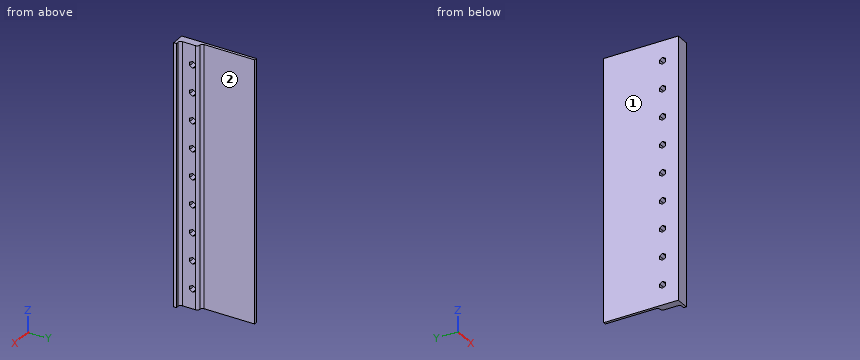
from build123d import *

# Parameters (mm, degrees)
GENERAL_EXTRUDE_DEPTH       = 925
ROUNDING_R                  = 5
ROLLER_HOLDERS_DEPTH        = 926.55388822
SKETCH5_W                   = 5
SKETCH5_H                   = 1850
GUARD_RAIL_DEPTH            = 100
GUARD_RAIL_SUPPORT_FILLET_R = 5
CUT_TO_SIZE_DEPTH           = 934.086276825
CUT_TO_SIZE_DEPTH_BACK      = 934.086276825
SKETCH6_W                   = 1357.48
SKETCH6_H                   = 140


with BuildPart() as part:
    # Sketch2 → General extrude (new, symmetric)
    with BuildSketch(Plane.XY):
        Polygon((-12.5, 20), (-12.5, -20), (12.5, -20), (12.5, -15), (2.5, -15), (2.5, 20), align=None)
    extrude(amount=GENERAL_EXTRUDE_DEPTH, both=True)

    # Rounding
    rounding_edges = [part.edges().sort_by_distance(p)[0] for p in [
        (2.5, 20, 0),
        (2.5, -15, 0),
    ]]
    fillet(rounding_edges, radius=ROUNDING_R)

    # Sketch3 → Roller holders (cut, through all)
    with BuildSketch(Plane.ZY.offset(12.5)):
        Polygon((-884.3762927, 3.8875), (-881.168390267, 9.44375), (-884.3762927, 15), (-890.792097567, 15), (-894, 9.44375), (-890.792097567, 3.8875), align=None)
        Polygon((-832.165457693, 3.8875), (-828.957555259, 9.44375), (-832.165457693, 15), (-838.581262559, 15), (-841.789164992, 9.44375), (-838.581262559, 3.8875), align=None)
        Polygon((-779.954622685, 3.8875), (-776.746720252, 9.44375), (-779.954622685, 15), (-786.370427551, 15), (-789.578329984, 9.44375), (-786.370427551, 3.8875), align=None)
        Polygon((-727.743787677, 3.8875), (-724.535885244, 9.44375), (-727.743787677, 15), (-734.159592543, 15), (-737.367494976, 9.44375), (-734.159592543, 3.8875), align=None)
        Polygon((-675.532952669, 3.8875), (-672.325050236, 9.44375), (-675.532952669, 15), (-681.948757535, 15), (-685.156659969, 9.44375), (-681.948757535, 3.8875), align=None)
        Polygon((-623.322117661, 3.8875), (-620.114215228, 9.44375), (-623.322117661, 15), (-629.737922528, 15), (-632.945824961, 9.44375), (-629.737922528, 3.8875), align=None)
        Polygon((-571.111282653, 3.8875), (-567.90338022, 9.44375), (-571.111282653, 15), (-577.52708752, 15), (-580.734989953, 9.44375), (-577.52708752, 3.8875), align=None)
        Polygon((-518.900447645, 3.8875), (-515.692545212, 9.44375), (-518.900447645, 15), (-525.316252512, 15), (-528.524154945, 9.44375), (-525.316252512, 3.8875), align=None)
        Polygon((-466.689612638, 3.8875), (-463.481710204, 9.44375), (-466.689612638, 15), (-473.105417504, 15), (-476.313319937, 9.44375), (-473.105417504, 3.8875), align=None)
        Polygon((-414.47877763, 3.8875), (-411.270875197, 9.44375), (-414.47877763, 15), (-420.894582496, 15), (-424.102484929, 9.44375), (-420.894582496, 3.8875), align=None)
        Polygon((-362.267942622, 3.8875), (-359.060040189, 9.44375), (-362.267942622, 15), (-368.683747488, 15), (-371.891649921, 9.44375), (-368.683747488, 3.8875), align=None)
        Polygon((-310.057107614, 3.8875), (-306.849205181, 9.44375), (-310.057107614, 15), (-316.47291248, 15), (-319.680814914, 9.44375), (-316.47291248, 3.8875), align=None)
        Polygon((-257.846272606, 3.8875), (-254.638370173, 9.44375), (-257.846272606, 15), (-264.262077472, 15), (-267.469979906, 9.44375), (-264.262077472, 3.8875), align=None)
        Polygon((-205.635437598, 3.8875), (-202.427535165, 9.44375), (-205.635437598, 15), (-212.051242465, 15), (-215.259144898, 9.44375), (-212.051242465, 3.8875), align=None)
        Polygon((-153.42460259, 3.8875), (-150.216700157, 9.44375), (-153.42460259, 15), (-159.840407457, 15), (-163.04830989, 9.44375), (-159.840407457, 3.8875), align=None)
        Polygon((-101.213767583, 3.8875), (-98.005865149, 9.44375), (-101.213767583, 15), (-107.629572449, 15), (-110.837474882, 9.44375), (-107.629572449, 3.8875), align=None)
        Polygon((-49.002932575, 3.8875), (-45.795030141, 9.44375), (-49.002932575, 15), (-55.418737441, 15), (-58.626639874, 9.44375), (-55.418737441, 3.8875), align=None)
        Polygon((3.207902433, 3.8875), (6.415804866, 9.44375), (3.207902433, 15), (-3.207902433, 15), (-6.415804866, 9.44375), (-3.207902433, 3.8875), align=None)
        Polygon((55.418737441, 3.8875), (58.626639874, 9.44375), (55.418737441, 15), (49.002932575, 15), (45.795030141, 9.44375), (49.002932575, 3.8875), align=None)
        Polygon((107.629572449, 3.8875), (110.837474882, 9.44375), (107.629572449, 15), (101.213767583, 15), (98.005865149, 9.44375), (101.213767583, 3.8875), align=None)
        Polygon((159.840407457, 3.8875), (163.04830989, 9.44375), (159.840407457, 15), (153.42460259, 15), (150.216700157, 9.44375), (153.42460259, 3.8875), align=None)
        Polygon((212.051242465, 3.8875), (215.259144898, 9.44375), (212.051242465, 15), (205.635437598, 15), (202.427535165, 9.44375), (205.635437598, 3.8875), align=None)
        Polygon((264.262077472, 3.8875), (267.469979906, 9.44375), (264.262077472, 15), (257.846272606, 15), (254.638370173, 9.44375), (257.846272606, 3.8875), align=None)
        Polygon((316.47291248, 3.8875), (319.680814914, 9.44375), (316.47291248, 15), (310.057107614, 15), (306.849205181, 9.44375), (310.057107614, 3.8875), align=None)
        Polygon((368.683747488, 3.8875), (371.891649921, 9.44375), (368.683747488, 15), (362.267942622, 15), (359.060040189, 9.44375), (362.267942622, 3.8875), align=None)
        Polygon((420.894582496, 3.8875), (424.102484929, 9.44375), (420.894582496, 15), (414.47877763, 15), (411.270875197, 9.44375), (414.47877763, 3.8875), align=None)
        Polygon((473.105417504, 3.8875), (476.313319937, 9.44375), (473.105417504, 15), (466.689612638, 15), (463.481710204, 9.44375), (466.689612638, 3.8875), align=None)
        Polygon((525.316252512, 3.8875), (528.524154945, 9.44375), (525.316252512, 15), (518.900447645, 15), (515.692545212, 9.44375), (518.900447645, 3.8875), align=None)
        Polygon((577.52708752, 3.8875), (580.734989953, 9.44375), (577.52708752, 15), (571.111282653, 15), (567.90338022, 9.44375), (571.111282653, 3.8875), align=None)
        Polygon((629.737922528, 3.8875), (632.945824961, 9.44375), (629.737922528, 15), (623.322117661, 15), (620.114215228, 9.44375), (623.322117661, 3.8875), align=None)
        Polygon((681.948757535, 3.8875), (685.156659969, 9.44375), (681.948757535, 15), (675.532952669, 15), (672.325050236, 9.44375), (675.532952669, 3.8875), align=None)
        Polygon((734.159592543, 3.8875), (737.367494976, 9.44375), (734.159592543, 15), (727.743787677, 15), (724.535885244, 9.44375), (727.743787677, 3.8875), align=None)
        Polygon((786.370427551, 3.8875), (789.578329984, 9.44375), (786.370427551, 15), (779.954622685, 15), (776.746720252, 9.44375), (779.954622685, 3.8875), align=None)
        Polygon((838.581262559, 3.8875), (841.789164992, 9.44375), (838.581262559, 15), (832.165457693, 15), (828.957555259, 9.44375), (832.165457693, 3.8875), align=None)
        Polygon((890.792097567, 3.8875), (894, 9.44375), (890.792097567, 15), (884.3762927, 15), (881.168390267, 9.44375), (884.3762927, 3.8875), align=None)
    extrude(amount=-ROLLER_HOLDERS_DEPTH, mode=Mode.SUBTRACT)

    # Sketch5 → Guard rail (add)
    with BuildSketch(Plane(origin=(0, 20, 0), x_dir=(1, 0, 0), z_dir=(0, 1, 0))):
        with Locations((-10, 0)):
            Rectangle(SKETCH5_W, SKETCH5_H)
    extrude(amount=GUARD_RAIL_DEPTH)

    # Guard rail support fillet
    guard_rail_support_fillet_edges = [part.edges().sort_by_distance(p)[0] for p in [
        (-7.5, 20, 0),
    ]]
    fillet(guard_rail_support_fillet_edges, radius=GUARD_RAIL_SUPPORT_FILLET_R - 0.0001)  # a hair under: the kernel refuses the full size

    # Sketch6 → CUT TO SIZE (cut, two sides: drawn at the far end of the back side and taken through both)
    with BuildSketch(Plane.ZY.offset(12.5).offset(-CUT_TO_SIZE_DEPTH_BACK)):
        with Locations((-246.26, 50)):
            Rectangle(SKETCH6_W, SKETCH6_H)
    extrude(amount=CUT_TO_SIZE_DEPTH + CUT_TO_SIZE_DEPTH_BACK, mode=Mode.SUBTRACT)


solid = part.part
Read the model definition and answer for the solid it produces. Units are mm, in the model's axes. Face numbers are marked on the shaded views. A direction names the side the tool comes from. Give positions to 0.01 mm unless a question says otherwise; leave off trailing zeros. Loops run counter-clockwise (first coordinate to the right, second up) from the corner with the lowest first, then second, coordinate; pieces in that order, holes last. Notation, with made-up numbers: M -36,-6.5 L 14,-6.5 A16 ccw 14,3.5 Z; hole C 50.5,34 d7. An arc over 180 degrees is marked long. Write each question's results on one line, items separated by ' | '.
1. Straight lines are drawn through the part: line 1 (Y direction, x = -1.75, z = 485); line 2 (Y direction, x = 7, z = 627.5); line 3 (X direction, y = -9, z = 600.5). For each, find the intervals that lie inside material, in ascending order. Write a range as [from, to].
Values:
line 1: y = [-20, 19.94] | line 2: y = [-20, -14.97] | line 3: x = [-12.5, 2.5]
2. Section C-C on y = 76.5 is taken. Give the vertices of the cut face in (x, z).
Values:
outline: M -12.5,432.48 L -7.5,432.48 L -7.5,925 L -12.5,925 Z
3. Section B-B on y = -4.5 is taken. Give the vertices of the cut face in (x, z).
Values:
outline: M -12.5,432.48 L 2.5,432.48 L 2.5,925 L -12.5,925 Z
4. Given pin 1 (5 mm diameter, centred on x = -2, z = 836, fed in from +Y); pin 2 (1.5 mm diameter, centred on x = 0, z = 570.5, fed in from +Y); pin 3 (1.9 mm diameter, centred on x = -1.5, z = 783, fed in from +Y); pin 4 (7 mm diameter, centred on x = -7, z = 886.5, fed in from +Y), each flat-ended and moving along its own axis, determine where each tip first touches the part or whether it passes through.
Values:
pin 1: stops at y = 20.42 | pin 2: stops at y = 19.68 | pin 3: stops at y = 20 | pin 4: stops at y = 120
5. A tool of negligible diameter and unlimited length cuts with its end or side. For the marked faces 1 and 2, from which of +Z, -Z, +X, -X, +Y, -Y can it reach the whole face along a straight path? Write none if from no direction.
Values:
face 1: +Z, -Z, -X, +Y, -Y | face 2: +Z, -Z, +X, +Y
